The listing builds one solid part. Answer for the finished solid, in the listing's coordinates (mm). A direction names the side the tool comes from. Round coordinates to 2 decimals unless told otherwise and drop trailing zeros. Order: outer loops, then holes, each group sorted by start corner. A loop starts at its lowest first (then second) coordinate and runs counter-clockwise, first axis right, second up. Notation, with made-up numbers: M 79,65.25 L 109,65.25 A20 cw 109,85.25 Z; hole C 39,-24.5 d6. An arc over 180 degrees is marked long. Write item = value, one per line. Start each with the question number.
(1) A cutting plane is placed at D-D, the plane x = 22. Determine the outline of the cut face in (y, z), and give its area (3 significant figures).
(2) Which of the six approach directions +Z, -Z, +X, -X, +Y, -Y give full straight-line access (tool end or side, diameter ignored) to faces 1 (the face through (15, -41, -77.065)), 2 (the face through (-13, -62, -19.677))?
(3) Each of these flat-tipped pins is pushed along its axis until it touches: pin 1 (6 mm diameter, centred on x = 7.5, z = -8.5, fed in from -Y); pin 2 (6 mm diameter, centred on y = -34, z = 3, fed in from +X). Where does it stop, or does it pass through?
(4) A cutting plane is placed at C-C, the plane z = 8. Determine the outline of the cut face in (x, y).
(5) A cutting plane is placed at B-B, the plane y = -16. Determine the outline of the cut face in (x, z).
(6) A cutting plane is placed at A-A, the plane x = -20. Determine the outline of the cut face in (y, z).
(7) Straight lines are drawn through the part: probe 1 along Z at (x, y) = (36, -43.5); probe 2 along Y at (x, z) = (-42, 2); probe 3 along X at (y, z) = (-27, 19.5). For each, find the intervals that lie inside material, in ascending order. Write a range as from..to.
from build123d import *

# Parameters (mm, degrees)
F0_W     = 156.905822
F0_H     = 108.593594
F1_DEPTH = 83.566
F3_DEPTH = 83.567
F4_W     = 43.500216
F4_H     = 51.205804
F5_DEPTH = 156.906822


with BuildPart() as f1:
    # F0 (on Front) → F1 (new body)
    with BuildSketch(Plane.XZ):
        with Locations((15.949223, -22.768164)):
            Rectangle(F0_W, F0_H)
    extrude(amount=F1_DEPTH)

    # F2 (on face) → F3 (cut, through all)
    with BuildSketch(Plane.XZ.offset(83.566)):
        Polygon((94.402134, 31.528633), (-13.758647, 31.528633), (94.402134, -77.064961), align=None)
    extrude(amount=-F3_DEPTH, mode=Mode.SUBTRACT)

    # F4 (on face) → F5 (cut, through all)
    with BuildSketch(Plane(origin=(-62.503688, 0, 0), x_dir=(0, -1, 0), z_dir=(-1, 0, 0))):
        with Locations((61.815892, 5.925731)):
            Rectangle(F4_W, F4_H)
    extrude(amount=-F5_DEPTH, mode=Mode.SUBTRACT)


solid = f1.part
Reported:
q1.outline = M -83.57,-77.06 L 0,-77.06 L 0,-4.37 L -40.07,-4.37 L -40.07,-19.68 L -83.57,-19.68 Z
q1.area = 5,410 mm²
q2.face_1 = -Z, +X, -X, +Y, -Y
q2.face_2 = +Z, +X, -X, -Y
q3.pin_1 = -40.07
q3.pin_2 = 17.64
q4.outline = M -62.5,-40.07 L 9.68,-40.07 L 9.68,0 L -62.5,0 Z
q5.outline = M -62.5,-77.06 L 94.4,-77.06 L -13.76,31.53 L -62.5,31.53 Z
q6.outline = M -83.57,-77.06 L 0,-77.06 L 0,31.53 L -40.07,31.53 L -40.07,-19.68 L -83.57,-19.68 Z
q7.probe_1 = -77.06..-19.68
q7.probe_2 = -40.07..0
q7.probe_3 = -62.5..-1.78
